from build123d import *

# Parameters (mm, degrees)
SKETCH1_R           = 12.7
BOSS_EXTRUDE1_DEPTH = 12.7
SKETCH2_R           = 6.35
CUT_EXTRUDE1_DEPTH  = 6.35
SKETCH3_R           = 2.778125
CUT_EXTRUDE2_DEPTH  = 20.05
FILLET1_R           = 1.27


with BuildPart() as part:
    # Sketch1 → Boss-Extrude1 (new body)
    with BuildSketch(Plane(origin=(0, 0, 0), x_dir=(1, 0, 0), z_dir=(0, 1, 0))):
        with Locations(Location((0, 0, 0), (0, 0, 270))):
            Circle(SKETCH1_R)
    extrude(amount=BOSS_EXTRUDE1_DEPTH)

    # Sketch2 → Cut-Extrude1 (cut)
    with BuildSketch(Plane(origin=(0, 12.7, 0), x_dir=(1, 0, 0), z_dir=(0, 1, 0))):
        with Locations(Location((0, 0, 0), (0, 0, 270))):
            Circle(SKETCH2_R)
    extrude(amount=-CUT_EXTRUDE1_DEPTH, mode=Mode.SUBTRACT)

    # Sketch3 → Cut-Extrude2 (cut, through all)
    with BuildSketch(Plane(origin=(0, 6.35, 0), x_dir=(1, 0, 0), z_dir=(0, 1, 0))):
        with Locations(Location((0, 0, 0), (0, 0, 270))):
            Circle(SKETCH3_R)
    extrude(amount=-CUT_EXTRUDE2_DEPTH, mode=Mode.SUBTRACT)

    # Fillet1
    fillet1_edges = [part.edges().sort_by_distance(p)[0] for p in [
        (0, 12.7, -12.7),
        (0, 12.7, -6.35),
    ]]
    fillet(fillet1_edges, radius=FILLET1_R)


solid = part.part
Here's how the part is built. I have some questions about the finished solid (model axes, mm). A direction names the side the tool comes from. Round coordinates to 2 decimals unless told otherwise and drop trailing zeros. Loops run counter-clockwise (first coordinate to the right, second up) from the corner with the lowest first, then second, coordinate; pieces in that order, holes last. Notation, with made-up numbers: (35.25, 65) -> (71.25, 65) arc R26 ccw to (71.25, 95) -> close; hole circle Ø8 at (32, 54). An arc over 180 degrees is marked (long way). Write each question's results on one line, items separated by ' | '.
(1) If I drill on L1, parallel to X at y = 4.75, z = 0; L2, parallel to Y at x = 1.5, z = -3; L3, parallel to X at y = 11.75, z = 1, over which ranges is the centre line in solid material (lowest first)?
Worked answers:
L1: -12.7 to -2.78, 2.78 to 12.7 | L2: 0 to 6.35 | L3: -12.62 to -6.31, 6.31 to 12.62
(2) For P1, Ø6.5, axis at x = 0, z = 0, coming from the -Y side; P2, Ø10, axis at x = -2.5, z = 0.5, coming from the +Y side; P3, Ø1, axis at x = -5, y = 5, coming from the -Z side; P4, Ø4, axis at x = 7, y = 11, coming from the -Z side, each with a flat end and sliding along its axis, tell me the tip position at first contact or that it passes through.
Worked answers:
P1: y = 0 | P2: y = 12.7 | P3: z = -11.88 | P4: z = -11.67
(3) If we section it at D-D, the plane y = 2.5: List the corners of the cut face in (x, z) for me.
Worked answers:
outline: circle Ø25.4 at (0, 0); hole circle Ø5.56 at (0, 0)
(4) If we section it at A-A, the plane z = 0: List the corners of the cut face in (x, y) for me, then the cut area to 3 significant figures.
Worked answers:
outline: (-12.7, 0) -> (-2.78, 0) -> (-2.78, 6.35) -> (-6.35, 6.35) -> (-6.35, 11.43) arc R1.27 ccw to (-7.62, 12.7) -> (-11.43, 12.7) arc R1.27 ccw to (-12.7, 11.43) -> close; (2.78, 0) -> (12.7, 0) -> (12.7, 11.43) arc R1.27 ccw to (11.43, 12.7) -> (7.62, 12.7) arc R1.27 ccw to (6.35, 11.43) -> (6.35, 6.35) -> (2.78, 6.35) -> close | area: 205 mm2
(5) If we section it at B-B, the plane x = 0: List the corners of the cut face in (y, z) for me, then the cut area to 3 significant figures.
Worked answers:
outline: (0, -12.7) -> (11.43, -12.7) arc R1.27 ccw to (12.7, -11.43) -> (12.7, -7.62) arc R1.27 ccw to (11.43, -6.35) -> (6.35, -6.35) -> (6.35, -2.78) -> (0, -2.78) -> close; (0, 2.78) -> (6.35, 2.78) -> (6.35, 6.35) -> (11.43, 6.35) arc R1.27 ccw to (12.7, 7.62) -> (12.7, 11.43) arc R1.27 ccw to (11.43, 12.7) -> (0, 12.7) -> close | area: 205 mm2
(6) If we section it at C-C, the plane y = 8.75: List the corners of the cut face in (x, z) for me, then the cut area to 3 significant figures.
Worked answers:
outline: circle Ø25.4 at (0, 0); hole circle Ø12.7 at (0, 0) | area: 380 mm2
(7) We'd pull the mould along Z, two halves only. Please class faces 3 (the face through (-7.5, 12.7, 2.4)), 4 (the face through (2.343, 3.219, 1.494)), 5 (the face through (-7.7, 5.6, -10.1)): released by +Z, released by -Z, zero draft, split by the parting line, or undercut.
Worked answers:
face 3: zero draft | face 4: undercut | face 5: split by the parting line
(8) For faces 1 (the face through (3, 0, 0)), 2 (the face through (-3.86, 8.93, -5.04)), which set-ups out of +Z, -Z, +X, -X, +Y, -Y let a thin tool reach every point of the face, with its end or its side?
Worked answers:
face 1: +Z, -Z, +X, -X, -Y | face 2: +Y
